CAD build for the part. Positions are in the model's coordinates, mm. Round coordinates to 2 decimals unless told otherwise and drop trailing zeros. Order: outer loops, then holes, each group sorted by start corner. A loop starts at its lowest first (then second) coordinate and runs counter-clockwise, first axis right, second up. Notation, with made-up numbers: (85, 63) - (131, 63) arc R5 ccw to (131, 72) - close; hole circle Ø7 at (-10, 26.25). An arc over 180 degrees is marked (long way). Use one line per item in the form item = value. Start each with the question number.
from build123d import *

# Parameters (mm, degrees)
BOSS_EXTRU_1_DEPTH      = 4
ENL_V_MAT_EXTRU_1_DEPTH = 74.295634249


with BuildPart() as part:
    # Esquisse1 → Boss.-Extru.1 (new body)
    with BuildSketch(Plane.XY):
        with BuildLine():
            Line((-6, -72.5), (6, -72.5))
            ThreePointArc((6, -72.5), (8.828427125, -71.328427125), (10, -68.5))
            Line((10, -68.5), (10, 68.5))
            ThreePointArc((10, 68.5), (8.828427125, 71.328427125), (6, 72.5))
            Line((6, 72.5), (-6, 72.5))
            ThreePointArc((-6, 72.5), (-8.828427125, 71.328427125), (-10, 68.5))
            Line((-10, 68.5), (-10, -68.5))
            ThreePointArc((-10, -68.5), (-8.828427125, -71.328427125), (-6, -72.5))
        make_face()
    extrude(amount=BOSS_EXTRU_1_DEPTH)

    # Esquisse2 → Enlèv. mat.-Extru.1 (cut, through all)
    with BuildSketch(Plane.XY.offset(4)):
        with BuildLine():
            Line((-2.5, -64), (-2.5, -56))
            ThreePointArc((-2.5, -56), (-2.207106781, -55.292893219), (-1.5, -55))
            Line((-1.5, -55), (1.5, -55))
            ThreePointArc((1.5, -55), (2.207106781, -55.292893219), (2.5, -56))
            Line((2.5, -56), (2.5, -64))
            ThreePointArc((2.5, -64), (2.207106781, -64.707106781), (1.5, -65))
            Line((1.5, -65), (-1.5, -65))
            ThreePointArc((-1.5, -65), (-2.207106781, -64.707106781), (-2.5, -64))
        make_face()
        with BuildLine():
            Line((-2.5, 56), (-2.5, 64))
            ThreePointArc((-2.5, 64), (-2.207106781, 64.707106781), (-1.5, 65))
            Line((-1.5, 65), (1.5, 65))
            ThreePointArc((1.5, 65), (2.207106781, 64.707106781), (2.5, 64))
            Line((2.5, 64), (2.5, 56))
            ThreePointArc((2.5, 56), (2.207106781, 55.292893219), (1.5, 55))
            Line((1.5, 55), (-1.5, 55))
            ThreePointArc((-1.5, 55), (-2.207106781, 55.292893219), (-2.5, 56))
        make_face()
    extrude(amount=-ENL_V_MAT_EXTRU_1_DEPTH, mode=Mode.SUBTRACT)


solid = part.part
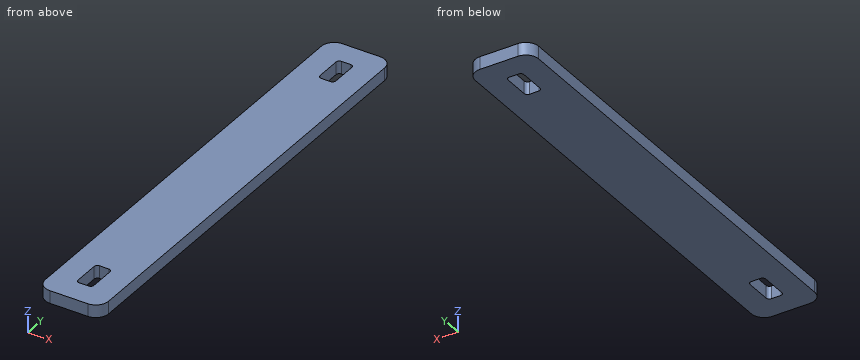
(1) Wall check: line 1 (Y direction, x = -0.5, z = 1.55); line 2 (Y direction, x = 2.25, z = 2.75); line 3 (X direction, y = -58, z = 1.1). Give the ranges that are in metal, low to high. Write a range as [from, to].
(2) Slice it at B-B (x = 8.75). Give the cut face in (y, z), and give its area (3 significant figures).
(3) Slice it at A-A (z = 1.5). Give the cut face in (x, y), and give its area (3 significant figures).
Results list:
q1.line_1 = [-72.5, -65], [-55, 55], [65, 72.5]
q1.line_2 = [-72.5, -64.66], [-55.34, 55.34], [64.66, 72.5]
q1.line_3 = [-10, -2.5], [2.5, 10]
q2.outline = (-71.4, 0) - (71.4, 0) - (71.4, 4) - (-71.4, 4) - close
q2.area = 571 mm²
q3.outline = (-10, -68.5) arc R4 ccw to (-6, -72.5) - (6, -72.5) arc R4 ccw to (10, -68.5) - (10, 68.5) arc R4 ccw to (6, 72.5) - (-6, 72.5) arc R4 ccw to (-10, 68.5) - close; hole (-2.5, -64) arc R1 ccw to (-1.5, -65) - (1.5, -65) arc R1 ccw to (2.5, -64) - (2.5, -56) arc R1 ccw to (1.5, -55) - (-1.5, -55) arc R1 ccw to (-2.5, -56) - close; hole (-2.5, 56) arc R1 ccw to (-1.5, 55) - (1.5, 55) arc R1 ccw to (2.5, 56) - (2.5, 64) arc R1 ccw to (1.5, 65) - (-1.5, 65) arc R1 ccw to (-2.5, 64) - close
q3.area = 2,790 mm²
